from build123d import *

# Parameters (mm, degrees)
ESQUISSE1_R             = 30
BOSS_EXTRU_1_DEPTH      = 17
ESQUISSE2_R             = 1.25
ENL_V_MAT_EXTRU_1_DEPTH = 100


with BuildPart() as part:
    # Esquisse1 → Boss.-Extru.1 (new body)
    with BuildSketch(Plane.XY):
        Circle(ESQUISSE1_R)
        with BuildLine():
            Line((0, 40), (0, 30))
            ThreePointArc((0, 30), (21.213203436, 21.213203436), (30, 0))
            Line((30, 0), (40, 0))
            ThreePointArc((40, 0), (28.284271247, 28.284271247), (0, 40))
        make_face()
        with BuildLine():
            ThreePointArc((0, -30), (-21.213203436, -21.213203436), (-30, 0))
            Line((-30, 0), (-40, 0))
            ThreePointArc((-40, 0), (-28.284271247, -28.284271247), (0, -40))
            Line((0, -40), (0, -30))
        make_face()
    extrude(amount=BOSS_EXTRU_1_DEPTH)

    # Esquisse2 → Enlèv. mat.-Extru.1 (cut)
    with BuildSketch(Plane.XY.offset(17)):
        Circle(ESQUISSE2_R)
    extrude(amount=-ENL_V_MAT_EXTRU_1_DEPTH, mode=Mode.SUBTRACT)


solid = part.part
Can you work these out from the model? Positions are in its coordinate system, mm. A direction names the side the tool comes from. Coordinates: 2 decimals unless noted, no trailing zeros. Loops run counter-clockwise (first coordinate to the right, second up) from the corner with the lowest first, then second, coordinate; pieces in that order, holes last. Notation, with made-up numbers: (79.25, -38) - (130.25, -38) arc R19 cw to (130.25, -13) - close; hole circle Ø2 at (25, -28.5). An arc over 180 degrees is marked (long way). Answer as a JSON object with one key per item and string values. Group by question number.
Item 1: If we section it at C-C (x = -33.5): List the corners of the cut face in (y, z) for me, plus the area to 3 significant figures.
Item 2: On a 3-axis mill with a long thin cutter (end or side, diameter ignored), from which of +Z, -Z, +X, -X, +Y, -Y can I reach the whole of each face in a straight line? I mean faces 1 (the face through (35, 0, 8)), 2 (the face through (0, 35, 8)), 3 (the face through (8, 1, 0)). Say none if no direction works.
Item 3: If I drill on L1, parallel to X at y = 12.5, z = 8.75; L2, parallel to X at y = -19.5, z = 12.25; L3, parallel to Y at x = 24, z = 13.75, over which ranges is the centre line in solid material (lowest first)? Write a range as from..to.
Item 4: If we section it at A-A (z = 2.25): List the corners of the cut face in (x, y) for me.
Item 5: If we mould it in two halves opening along X, with no side actions, what happens to faces 4 (the face through (-20.979, 21.445, 8.381)), 5 (the face through (-35, 0, 8)), 6 (the face through (-0.27, -1.22, 8.62))? For each: released by +X, released by -X, zero draft, split by the parting line, or undercut.
Item 6: For pin 1 (5 mm diameter, centred on x = 14.5, z = 4.5, fed in from -Y); pin 2 (5 mm diameter, centred on y = -12, z = 11, fed in from -X); pin 3 (1.5 mm diameter, centred on x = -29, z = 5.5, fed in from -Y), each with a flat end and sliding along its axis, tell me the tip position at first contact or that it passes through.
Item 7: If we section it at B-B (y = 6): List the corners of the cut face in (x, z) for me, plus the area to 3 significant figures.
Returned:
{
 "1": {"outline": "(-21.86, 0) - (0, 0) - (0, 17) - (-21.86, 17) - close", "area": "372 mm²"},
 "2": {"face 1": "+Z, -Z, +X, -Y", "face 2": "+Z, -Z, -X, +Y", "face 3": "-Z, +X, -X, +Y, -Y"},
 "3": {"L1": "x = -27.27..38", "L2": "x = -34.92..22.8", "L3": "y = -18..32"},
 "4": {"outline": "(-40, 0) arc R40 ccw to (0, -40) - (0, -30) arc R30 ccw to (30, 0) - (40, 0) arc R40 ccw to (0, 40) - (0, 30) arc R30 ccw to (-30, 0) - close; hole circle Ø2.5 at (0, 0)"},
 "5": {"face 4": "released by -X", "face 5": "zero draft", "face 6": "undercut"},
 "6": {"pin 1": "stops at y = -27.5", "pin 2": "stops at x = -38.86", "pin 3": "stops at y = -28.32"},
 "7": {"outline": "(-29.39, 0) - (39.55, 0) - (39.55, 17) - (-29.39, 17) - close", "area": "1,170 mm²"}
}
